Can you work these out from the drawing? Everything is in mm from the part's minimum corner. Round coordinates to 2 decimals unless told otherwise and drop trailing zeros. Order: outer loops, then holes, each group sorted by start corner. A loop starts at its lowest first (then second) coordinate and runs counter-clockwise, first axis right, second up. Notation, with made-up numbers: (54.25, -37.5) - (74.25, -37.5) arc R15 cw to (74.25, -17.5) - close; hole circle Ø6 at (11, 4.5). An arc over 180 degrees is marked (long way). Answer as a JSON object with one key per item and string values.
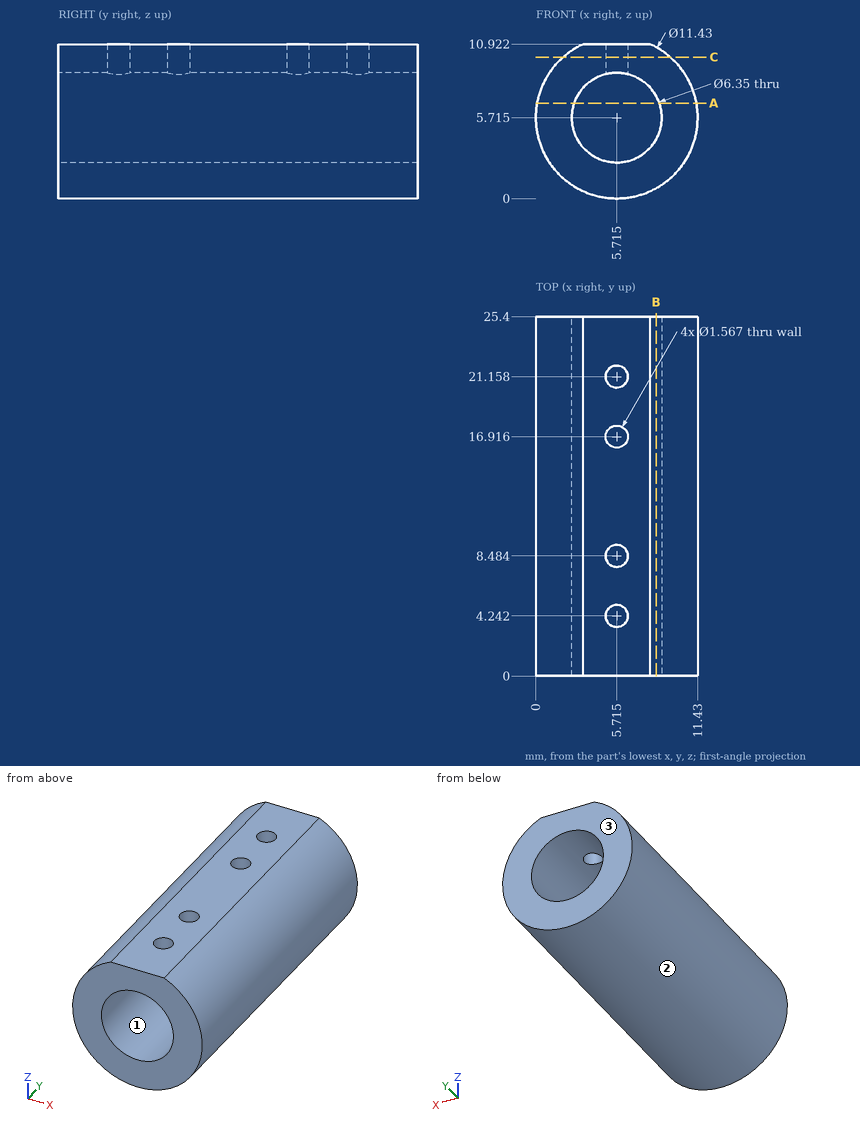
1. If I drill on L1, parallel to Y at x = 5.75, z = 9.25 (1 decimal); L2, parallel to Z at x = 5.5, y = 22.25; L3, parallel to Z at x = 5, y = 2.75 (1 decimal), over which ranges is the centre line in solid material (lowest first)? Write a range as [from, to].
Responses:
{"L1": "[0, 3.5], [5, 7.7], [9.3, 16.1], [17.7, 20.4], [21.9, 25.4]", "L2": "[0, 2.55], [8.88, 10.92]", "L3": "[0, 2.6], [8.8, 10.9]"}
2. Thinking about a two-plate mould opening in X: for the marked faces 1, 2 and 3, which applies, pulls with the +X half, pulls with the -X half, needs draft (parallel to the pull), parting line crosses it, or undercut?
Responses:
{"face 1": "undercut", "face 2": "parting line crosses it", "face 3": "needs draft"}
3. Imagine slicing it at A-A (z = 6.75). List the corners of the cut face in (x, y) for me (1 decimal).
Responses:
{"outline": "(0.1, 0) - (2.7, 0) - (2.7, 25.4) - (0.1, 25.4) - close; (8.7, 0) - (11.3, 0) - (11.3, 25.4) - (8.7, 25.4) - close"}
4. Imagine slicing it at C-C (z = 10). List the corners of the cut face in (x, y) for me (1 decimal).
Responses:
{"outline": "(1.9, 0) - (9.5, 0) - (9.5, 25.4) - (1.9, 25.4) - close; hole circle Ø1.6 at (5.7, 4.2); hole circle Ø1.6 at (5.7, 8.5); hole circle Ø1.6 at (5.7, 16.9); hole circle Ø1.6 at (5.7, 21.2)"}
5. Imagine slicing it at B-B (x = 8.5). List the corners of the cut face in (y, z) for me (1 decimal), plus the area to 3 significant figures.
Responses:
{"outline": "(0, 0.7) - (25.4, 0.7) - (25.4, 4.2) - (0, 4.2) - close; (0, 7.2) - (25.4, 7.2) - (25.4, 10.7) - (0, 10.7) - close", "area": "176 mm2"}
6. For P1, Ø1.3, axis at x = 5.72, y = 4.24, coming from the +Z side, with a flat end and sliding along its axis, tell me the tip position at first contact or that it passes through.
Responses:
{"P1": "z = 2.61"}
